Design review of the part built by this model. Coordinates are the model's own, in mm. Face numbers are marked on the shaded views. Coordinates: 2 decimals unless noted, no trailing zeros. Loops run counter-clockwise (first coordinate to the right, second up) from the corner with the lowest first, then second, coordinate; pieces in that order, holes last. Notation, with made-up numbers: (-22.75, 72) -> (-7.75, 72) arc R15 ccw to (-7.75, 78) -> close; hole circle Ø4 at (4, 48.25). An arc over 180 degrees is marked (long way). Answer in a Markdown table with one row per item.
```python
from build123d import *

# Parameters (mm, degrees)
SKETCH1_R           = 4
BOSS_EXTRUDE1_DEPTH = 25
SKETCH2_R           = 2.475
CUT_EXTRUDE1_DEPTH  = 15
SKETCH4_R           = 3.5052
BOSS_EXTRUDE2_DEPTH = 15


with BuildPart() as part:
    # Sketch1 → Boss-Extrude1 (new body)
    with BuildSketch(Plane(origin=(0, 0, 0), x_dir=(0, 0, -1), z_dir=(1, 0, 0))):
        Circle(SKETCH1_R)
    extrude(amount=BOSS_EXTRUDE1_DEPTH)

    # Sketch2 → Cut-Extrude1 (cut)
    with BuildSketch(Plane(origin=(0, 0, 0), x_dir=(0, 0, -1), z_dir=(1, 0, 0))):
        Circle(SKETCH2_R)
    extrude(amount=CUT_EXTRUDE1_DEPTH, mode=Mode.SUBTRACT)

    # Sketch4 → Boss-Extrude2 (add)
    with BuildSketch(Plane(origin=(25, 0, 0), x_dir=(0, 0, -1), z_dir=(1, 0, 0))):
        Circle(SKETCH4_R)
    extrude(amount=BOSS_EXTRUDE2_DEPTH)


solid = part.part
```
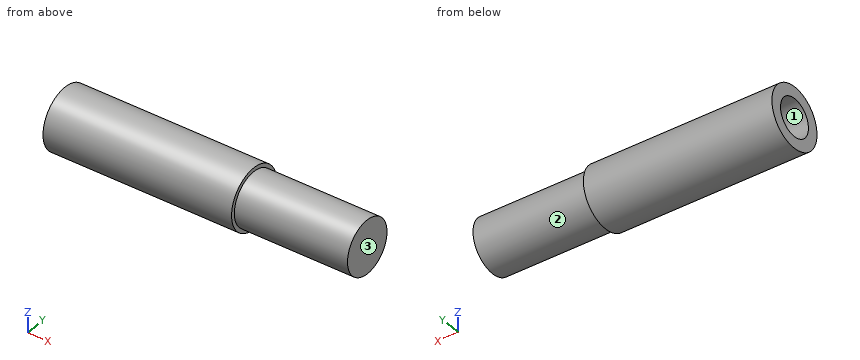
(1) Draft analysis for pull direction Y (two halves, no side actions). For the marked faces 1, 2 and 3, state which applies: pulls with the +Y half, pulls with the -Y half, needs draft (parallel to the pull), parting line crosses it, or undercut.
Evaluation:
| item | result |
|---|---|
| face 1 | undercut |
| face 2 | parting line crosses it |
| face 3 | needs draft |
(2) To check wall thickness, follow probe 1 along Y at (x, z) = (9, 0) (3 decimals); probe 2 along X at (y, z) = (-1.5, 0.25); probe 3 along Z at (x, y) = (13, 1). State the ranges of each line that lie inside material, in increasing order.
Evaluation:
| item | result |
|---|---|
| probe 1 | y = -4 to -2.475, 2.475 to 4 |
| probe 2 | x = 15 to 40 |
| probe 3 | z = -3.87 to -2.26, 2.26 to 3.87 |
(3) Take a section at D-D on z = 3. Give the boundary of the cut face in (x, y).
Evaluation:
| item | result |
|---|---|
| outline | (0, -2.65) -> (25, -2.65) -> (25, -1.81) -> (40, -1.81) -> (40, 1.81) -> (25, 1.81) -> (25, 2.65) -> (0, 2.65) -> close |
(4) Take a section at A-A on z = 0. Give the boundary of the cut face in (x, y) (3 decimals).
Evaluation:
| item | result |
|---|---|
| outline | (0, -4) -> (25, -4) -> (25, -3.505) -> (40, -3.505) -> (40, 3.505) -> (25, 3.505) -> (25, 4) -> (0, 4) -> (0, 2.475) -> (15, 2.475) -> (15, -2.475) -> (0, -2.475) -> close |
(5) For pin 1 (1 mm diameter, centred on x = 26.5, y = -1, fed in from -Z); pin 2 (1.5 mm diameter, centred on x = 19.5, z = -2.5, fed in from -Y); pin 3 (1.5 mm diameter, centred on x = 5, z = -1, fed in from -Y), all flat-tipped, find the tip position at first contact; note any pin that passes through.
Evaluation:
| item | result |
|---|---|
| pin 1 | stops at z = -3.47 |
| pin 2 | stops at y = -3.6 |
| pin 3 | stops at y = -3.99 |
(6) Take a section at B-B on y = 0.5. Give the boundary of the cut face in (x, z).
Evaluation:
| item | result |
|---|---|
| outline | (0, -3.97) -> (25, -3.97) -> (25, -3.47) -> (40, -3.47) -> (40, 3.47) -> (25, 3.47) -> (25, 3.97) -> (0, 3.97) -> (0, 2.42) -> (15, 2.42) -> (15, -2.42) -> (0, -2.42) -> close |
(7) Take a section at C-C on x = 35. Give the boundary of the cut face in (y, z), and give its area (3 significant figures).
Evaluation:
| item | result |
|---|---|
| outline | circle Ø7.01 at (0, 0) |
| area | 38.6 mm² |
